Here's how the part is built. I have some questions about the finished solid (model axes, mm). Coordinates: 2 decimals unless noted, no trailing zeros. Write each loop counter-clockwise with the first axis right and the second up, starting at its lowest first coordinate (ties: lowest second). Pieces come first, ordered by that corner, then holes.
(1) For pin 1 Ø1.8 at (x, y) = (-8, 25) entering from +Z, with a flat end and sliding along its axis, tell me the tip position at first contact or that it passes through.
(2) Imagine slicing it at C-C, the plane y = -8. List the corners of the cut face in (x, z) for me, plus the area to 3 significant figures.
(3) Imagine slicing it at B-B, the plane x = -8. List the corners of the cut face in (y, z) for me, plus the area to 3 significant figures.
(4) Imagine slicing it at D-D, the plane x = -14.5. List the corners of the cut face in (y, z) for me, plus the area to 3 significant figures.
(5) Imagine slicing it at A-A, the plane y = 18. List the corners of the cut face in (x, z) for me.
(6) Please list where these lines run through material, in increasing order: probe 1 along Y at (x, z) = (-8, 0.7); probe 2 along Y at (x, z) = (14.5, 2.3); probe 3 along Y at (x, z) = (5, 1).
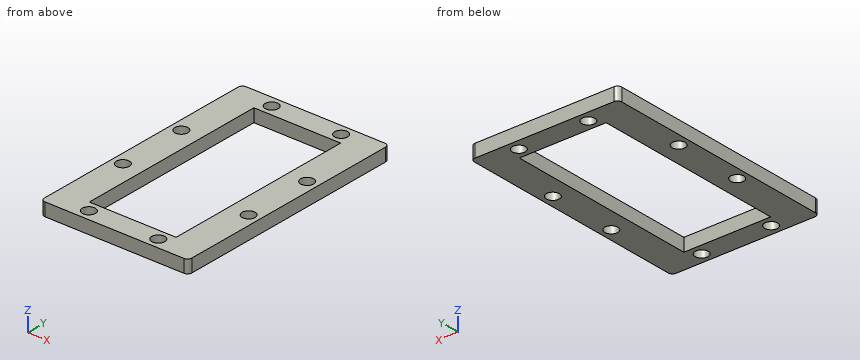
```python
from build123d import *

# Parameters (mm, degrees)
F0_W     = 34
F0_H     = 55
F0_R     = 1.5
F0_W_2   = 20
F0_H_2   = 45
F1_DEPTH = 3
F2_R     = 1.5
F3_DEPTH = 5
F4_R     = 1


with BuildPart() as f1:
    # F0 (on Top) → F1 (new body)
    with BuildSketch(Plane.XY):
        Rectangle(F0_W, F0_H)
        with Locations((-8, -25)):
            Circle(F0_R, mode=Mode.SUBTRACT)
        with Locations((8, -25)):
            Circle(F0_R, mode=Mode.SUBTRACT)
        with Locations((-8, 25)):
            Circle(F0_R, mode=Mode.SUBTRACT)
        Rectangle(F0_W_2, F0_H_2, mode=Mode.SUBTRACT)
        with Locations((8, 25)):
            Circle(F0_R, mode=Mode.SUBTRACT)
    extrude(amount=F1_DEPTH)

    # F2 (on face) → F3 (cut)
    with BuildSketch(Plane.XY.offset(3)):
        with Locations((-14.5, 8)):
            Circle(F2_R)
        with Locations((14.5, 8)):
            Circle(F2_R)
        with Locations((-14.5, -8)):
            Circle(F2_R)
        with Locations((14.5, -8)):
            Circle(F2_R)
    extrude(amount=-F3_DEPTH, mode=Mode.SUBTRACT)

    # F4
    f4_edges = [f1.edges().sort_by_distance(p)[0] for p in [
        (-17, 27.5, 1.5),
        (17, 27.5, 1.5),
        (17, -27.5, 1.5),
        (-17, -27.5, 1.5),
    ]]
    fillet(f4_edges, radius=F4_R)


solid = f1.part
```
Recorded:
1. pin 1: passes through
2. outline: (-17, 0) - (-16, 0) - (-16, 3) - (-17, 3) - close; (-13, 0) - (-10, 0) - (-10, 3) - (-13, 3) - close; (10, 0) - (13, 0) - (13, 3) - (10, 3) - close; (16, 0) - (17, 0) - (17, 3) - (16, 3) - close
2. area: 24.0 mm2
3. outline: (-27.5, 0) - (-26.5, 0) - (-26.5, 3) - (-27.5, 3) - close; (-23.5, 0) - (-22.5, 0) - (-22.5, 3) - (-23.5, 3) - close; (22.5, 0) - (23.5, 0) - (23.5, 3) - (22.5, 3) - close; (26.5, 0) - (27.5, 0) - (27.5, 3) - (26.5, 3) - close
3. area: 12.0 mm2
4. outline: (-27.5, 0) - (-9.5, 0) - (-9.5, 3) - (-27.5, 3) - close; (-6.5, 0) - (6.5, 0) - (6.5, 3) - (-6.5, 3) - close; (9.5, 0) - (27.5, 0) - (27.5, 3) - (9.5, 3) - close
4. area: 147 mm2
5. outline: (-17, 0) - (-10, 0) - (-10, 3) - (-17, 3) - close; (10, 0) - (17, 0) - (17, 3) - (10, 3) - close
6. probe 1: y = -27.5 to -26.5, -23.5 to -22.5, 22.5 to 23.5, 26.5 to 27.5
6. probe 2: y = -27.5 to -9.5, -6.5 to 6.5, 9.5 to 27.5
6. probe 3: y = -27.5 to -22.5, 22.5 to 27.5
